from build123d import *

# Parameters (mm, degrees)
F0_W     = 685.8
F0_H     = 203.2
F1_DEPTH = 19.05
F2_SIZE  = 6.35
F3_SIZE  = 6.35


with BuildPart() as f1:
    # F0 (on Top) → F1 (new body)
    with BuildSketch(Plane.XY):
        with Locations((-124.934961, 0.697705)):
            Rectangle(F0_W, F0_H)
    extrude(amount=F1_DEPTH)

    # F2
    f2_edges = [f1.edges().sort_by_distance(p)[0] for p in [
        (217.965039, 0.697705, 19.05),
        (-124.934961, 102.297705, 19.05),
        (-467.834961, 0.697705, 19.05),
        (-124.934961, -100.902295, 19.05),
    ]]
    chamfer(f2_edges, length=F2_SIZE)

    # F3
    f3_edges = [f1.edges().sort_by_distance(p)[0] for p in [
        (217.965039, 0.697705, 0),
        (-124.934961, 102.297705, 0),
        (-467.834961, 0.697705, 0),
        (-124.934961, -100.902295, 0),
    ]]
    chamfer(f3_edges, length=F3_SIZE)


solid = f1.part
Here's how the part is built. I have some questions about the finished solid (model axes, mm). Coordinates: 2 decimals unless noted, no trailing zeros. Write each loop counter-clockwise with the first axis right and the second up, starting at its lowest first coordinate (ties: lowest second). Pieces come first, ordered by that corner, then holes.
Item 1: I want a section at B-B on z = 15.75. Write out the boundary of the cut face in (x, y).
Item 2: I want a section at A-A on x = -391. Write out the boundary of the cut face in (y, z), and give its area (3 significant figures).
Item 3: If I drill on line 1 (X direction, y = 27, z = 15.5); line 2 (Y direction, x = -369, z = 14.75); line 3 (X direction, y = 26, z = 1), over which ranges is the centre line in solid material (lowest first)?
Item 4: Will these pins go through, and if not, where does the flat tip stop? pin 1 (8 mm diameter, centred on y = -41, z = 15, fed in from +X); pin 2 (1 mm diameter, centred on y = 46, z = 3.5, fed in from -X).
Findings below:
1. outline: (-464.78, -97.85) - (214.92, -97.85) - (214.92, 99.25) - (-464.78, 99.25) - close
2. outline: (-100.9, 6.35) - (-94.55, 0) - (95.95, 0) - (102.3, 6.35) - (102.3, 12.7) - (95.95, 19.05) - (-94.55, 19.05) - (-100.9, 12.7) - close
2. area: 3,790 mm2
3. line 1: x = -465.03 to 215.17
3. line 2: y = -98.85 to 100.25
3. line 3: x = -462.48 to 212.62
4. pin 1: stops at x = 217.97
4. pin 2: stops at x = -465.48
